Part model, mm, in its own coordinate system. A direction names the side the tool comes from. Coordinates: 2 decimals unless noted, no trailing zeros. Loops run counter-clockwise (first coordinate to the right, second up) from the corner with the lowest first, then second, coordinate; pieces in that order, holes last. Notation, with made-up numbers: M -27.5,35.25 L 8.5,35.25 A19 cw 8.5,68.25 Z; hole C -21.75,42.25 d8. An arc over 180 degrees is marked long. Answer as a JSON object with one key per item and string values. Group by question number.
1. Saw through at C-C on x = 51. Write the cut outline in (y, z).
2. 3-axis set-ups, long thin cutter, end or side, ignore diameter. For faces 5 (the face through (-25, 2.36, 20)), 6 (the face through (-67.54, 20.59, 40.14)), 7 (the face through (-65, 6, 30)), 8 (the face through (42, 0, 3)): which of +Z, -Z, +X, -X, +Y, -Y reach the whole face in a straight line?
3. Saw through at D-D on y = 0. Write the cut outline in (x, z), then the cut area to 3 significant figures.
4. Drill centre lines: L1, parallel to Z at x = -67.55, y = 19; L2, parallel to Y at x = -3, z = 1.2; L3, parallel to X at y = 8, z = 27. Where is each one in solid material? Low to high.
5. Saw through at B-B on z = 20. Write the cut outline in (x, y) (3 decimals), then the cut area to 3 significant figures.
6. Saw through at A-A on y = 15.5. Write the cut outline in (x, z).
7. Drop flat-ended pins along their axis: pin 1 Ø6.5 at (y, z) = (19, 20) entering from +X; pin 2 Ø4 at (x, y) = (38, -14) entering from +Z; pin 3 Ø17 at (x, y) = (23, 3.5) entering from +Z (3 decimals). Give the stop position or say it passes through.
8. Mould opens along Z. For faces 1 (the face through (-67.535, 26.289, 48.196)), 2 (the face through (-67.54, -17.41, 40.14)), 3 (the face through (-68, 19, 22)), 4 (the face through (-70, 0, 25)) say: released by +Z, released by -Z, zero draft, split by the parting line, or undercut.
from build123d import *

# Parameters (mm, degrees)
F1_DEPTH = 50
F0_R     = 2
F0_R_2   = 9
F2_DEPTH = 5
F3_R     = 6
F4_DEPTH = 1
F0_W     = 105
F0_H     = 5
F5_DEPTH = 45
F7_DEPTH = 25
F8_R     = 2
F9_DEPTH = 25


with BuildPart() as f1:
    # F0 (on Top) → F1 (new body)
    with BuildSketch(Plane.XY):
        Polygon((-70, -28), (-65, -28), (-65, -2.640025), (-65, 2.359975), (-65, 28), (-70, 28), align=None)
    extrude(amount=F1_DEPTH)

    # F0 (on Top) → F2 (join)
    with BuildSketch(Plane.XY):
        Polygon((-65, -28), (65, -28), (65, 28), (-65, 28), (-65, 2.359975), (40, 2.359975), (40, -2.640025), (-65, -2.640025), align=None)
        with Locations((-31.100778, -22)):
            Circle(F0_R, mode=Mode.SUBTRACT)
        with Locations((-3, -22)):
            Circle(F0_R, mode=Mode.SUBTRACT)
        with Locations((-31.100778, 22)):
            Circle(F0_R, mode=Mode.SUBTRACT)
        with Locations((-3, 22)):
            Circle(F0_R, mode=Mode.SUBTRACT)
        with Locations((51, 0)):
            Circle(F0_R_2, mode=Mode.SUBTRACT)
    extrude(amount=F2_DEPTH)

    # F3
    f3_edges = [f1.edges().sort_by_distance(p)[0] for p in [
        (-67.5, 28, 50),
        (-67.5, -28, 50),
        (65, -28, 2.5),
        (65, 28, 2.5),
        (-65, -15.320012, 5),
        (-65, 15.179988, 5),
    ]]
    fillet(f3_edges, radius=F3_R)

    # F0 (on Top) → F4 (join)
    with BuildSketch(Plane.XY):
        with Locations((51, 0)):
            Circle(F0_R_2)
    extrude(amount=F4_DEPTH)

    # F0 (on Top) → F5 (join)
    with BuildSketch(Plane.XY):
        with Locations((-12.5, -0.140025)):
            Rectangle(F0_W, F0_H)
    extrude(amount=F5_DEPTH)

    # F6 (on face) → F7 (cut)
    with BuildSketch(Plane.XZ.offset(2.640025)):
        Polygon((40, 45), (-65, 45), (40, 5), align=None)
    extrude(amount=-F7_DEPTH, mode=Mode.SUBTRACT)

    # F8 (on face) → F9 (cut)
    with BuildSketch(Plane(origin=(-70, 0, 0), x_dir=(0, -1, 0), z_dir=(-1, 0, 0))):
        with Locations((-19, 41.354249)):
            Circle(F8_R)
        with Locations((-19, 20)):
            Circle(F8_R)
        with Locations((19, 41.354249)):
            Circle(F8_R)
        with Locations((19, 20)):
            Circle(F8_R)
    extrude(amount=-F9_DEPTH, mode=Mode.SUBTRACT)


solid = f1.part
Outcome:
{
 "1": {"outline": "M -28,0 L 28,0 L 28,5 L 9,5 L 9,1 L -9,1 L -9,5 L -28,5 Z"},
 "2": {"face 5": "+Z, +X, +Y", "face 6": "+X, -X", "face 7": "+Z, +X", "face 8": "+Z"},
 "3": {"outline": "M -70,0 L 65,0 L 65,5 L 60,5 L 60,1 L 42,1 L 42,5 L 40,5 L -65,45 L -65,50 L -70,50 Z", "area": "2,930 mm²"},
 "4": {"L1": "z = 0 to 18, 22 to 39.35, 43.35 to 50", "L2": "y = -28 to -24, -20 to 20, 24 to 28", "L3": "x = -70 to -65"},
 "5": {"outline": "M -70,-28 L -65,-28 L -65,-21 L -70,-21 Z; M -70,-17 L -65,-17 L -65,-2.64 L 0.625,-2.64 L 0.625,2.36 L -65,2.36 L -65,17 L -70,17 Z; M -70,21 L -65,21 L -65,28 L -70,28 Z", "area": "568 mm²"},
 "6": {"outline": "M -70,0 L 65,0 L 65,5 L -59,5 A6 cw -65,11 L -65,50 L -70,50 Z"},
 "7": {"pin 1": "stops at x = -65", "pin 2": "stops at z = 5", "pin 3": "stops at z = 14.685"},
 "8": {"face 1": "released by +Z", "face 2": "undercut", "face 3": "undercut", "face 4": "zero draft"}
}
